Part model, mm, in its own coordinate system. Face numbers are marked on the shaded views. A direction names the side the tool comes from. Round coordinates to 2 decimals unless told otherwise and drop trailing zeros. Write each loop counter-clockwise with the first axis right and the second up, starting at its lowest first coordinate (ties: lowest second). Pieces come first, ordered by that corner, then holes.
1) Saw through at D-D on z = 0. Count the separate pieces of the cut face and the enclosed holes in it, and give its area (3 significant figures).
2) Flat gauge pins, fed straight in: pin 1 (3 mm diameter, centred on x = 20.5, z = -12, fed in from +Y); pin 2 (9.5 mm diameter, centred on x = 39, z = 0, fed in from +Y); pin 3 (8 mm diameter, centred on x = -6.5, z = 16, fed in from +Y); pin 4 (1 mm diameter, centred on y = -10, z = -17.5, fed in from +X). Where does each tip first touch, or does it go through?
3) Saw through at C-C on y = -13.5. Write the cut outline in (x, z).
4) Saw through at A-A on x = 0. Write the cut outline in (y, z) (3 decimals).
5) Which spindle directions (+Z, -Z, +X, -X, +Y, -Y) get a long thin tool onto all of the face, cutting with end or side? Do the marked faces 1, 2, 3 and 4. Say none if no direction does.
6) Pull direction Z, two halves, no side cores. Call the marked faces 5, 6 and 7: +Z half, -Z half, draft (parallel to the pull), parting line (faces both ways), or undercut.
7) Saw through at B-B on y = -5.5. Write the cut outline in (x, z).
8) Drill centre lines: L1, parallel to X at y = -4, z = 0; L2, parallel to Z at x = 0, y = 9; L3, parallel to Z at x = 0, y = -3. Where is each one in solid material? Low to high.
```python
from build123d import *

# Parameters (mm, degrees)
BOSS_EXTRUDE1_DEPTH = 23
CUT_EXTRUDE1_DEPTH  = 46
SKETCH4_R           = 6
CUT_EXTRUDE2_DEPTH  = 46
CUT_EXTRUDE3_DEPTH  = 46
SKETCH6_R           = 4
CUT_EXTRUDE4_DEPTH  = 16
SKETCH7_R           = 3
CUT_EXTRUDE5_DEPTH  = 71.608515808


with BuildPart() as part:
    # Sketch1 → Boss-Extrude1 (new, symmetric)
    with BuildSketch(Plane.XY):
        with BuildLine():
            Line((-54, 3.825), (-30.877783275, 3.825))
            ThreePointArc((-30.877783275, 3.825), (0, 15.075), (30.877783275, 3.825))
            Line((30.877783275, 3.825), (54, 3.825))
            Line((54, 3.825), (54, -8.175))
            Line((54, -8.175), (28, -8.175))
            Line((28, -8.175), (28, -24.175))
            Line((28, -24.175), (22.348098353, -24.175))
            ThreePointArc((22.348098353, -24.175), (0, -8.925), (-22.348098353, -24.175))
            Line((-22.348098353, -24.175), (-28, -24.175))
            Line((-28, -24.175), (-28, -8.175))
            Line((-28, -8.175), (-54, -8.175))
            Line((-54, -8.175), (-54, 3.825))
        make_face()
    extrude(amount=BOSS_EXTRUDE1_DEPTH, both=True)

    # Sketch2 → Cut-Extrude1 (cut)
    with BuildSketch(Plane(origin=(0, 3.825, 0), x_dir=(1, 0, 0), z_dir=(0, 1, 0))):
        with BuildLine():
            ThreePointArc((48.856934001, -23), (54, 0), (48.856934001, 23))
            Line((48.856934001, 23), (54, 23))
            Line((54, 23), (85.001299568, 23))
            Line((85.001299568, 23), (85.001299568, -23))
            Line((85.001299568, -23), (54, -23))
            Line((54, -23), (48.856934001, -23))
        make_face()
        with BuildLine():
            Line((-48.856934001, 23), (-68.265292399, 23))
            Line((-68.265292399, 23), (-68.265292399, -23))
            Line((-68.265292399, -23), (-54, -23))
            Line((-54, -23), (-48.856934001, -23))
            ThreePointArc((-48.856934001, -23), (-54, 0), (-48.856934001, 23))
        make_face()
    extrude(amount=-CUT_EXTRUDE1_DEPTH, mode=Mode.SUBTRACT)

    # Sketch4 → Cut-Extrude2 (cut)
    with BuildSketch(Plane(origin=(0, 3.825, 0), x_dir=(1, 0, 0), z_dir=(0, 1, 0))):
        with Locations(Location((-39, 0, 0), (0, 0, 270))):
            Circle(SKETCH4_R)
        with Locations(Location((39, 0, 0), (0, 0, 270))):
            Circle(SKETCH4_R)
    extrude(amount=-CUT_EXTRUDE2_DEPTH, mode=Mode.SUBTRACT)

    # Sketch5 → Cut-Extrude3 (cut)
    with BuildSketch(Plane(origin=(0, 3.825, 0), x_dir=(1, 0, 0), z_dir=(0, 1, 0))):
        with BuildLine():
            Line((-30.877783275, 13.785122251), (-30.877783275, -13.785122251))
            ThreePointArc((-30.877783275, -13.785122251), (-23, 0), (-30.877783275, 13.785122251))
        make_face()
        with BuildLine():
            Line((30.877783275, 13.785122251), (30.877783275, -13.785122251))
            ThreePointArc((30.877783275, -13.785122251), (23, 0), (30.877783275, 13.785122251))
        make_face()
    extrude(amount=CUT_EXTRUDE3_DEPTH, mode=Mode.SUBTRACT)

    # Sketch6 → Cut-Extrude4 (cut)
    with BuildSketch(Plane(origin=(0, 15.075, 0), x_dir=(1, 0, 0), z_dir=(0, 1, 0))):
        with Locations(Location((0, 0, 0), (0, 0, 270))):
            Circle(SKETCH6_R)
    extrude(amount=-CUT_EXTRUDE4_DEPTH, mode=Mode.SUBTRACT)

    # Sketch7 → Cut-Extrude5 (cut, through all)
    with BuildSketch(Plane(origin=(0, 15.075, 0), x_dir=(1, 0, 0), z_dir=(0, 1, 0))):
        with Locations(Location((0, 0, 0), (0, 0, 270))):
            Circle(SKETCH7_R)
    extrude(amount=-CUT_EXTRUDE5_DEPTH, mode=Mode.SUBTRACT)


solid = part.part
```
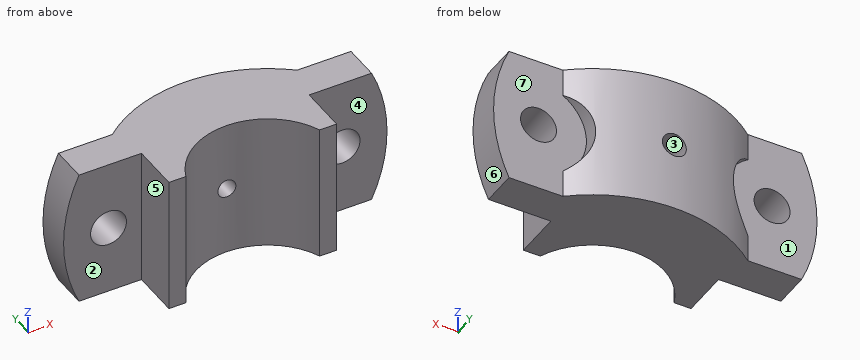
Completed:
1. separate pieces: 4
1. enclosed holes: 0
1. area: 1,660 mm2
2. pin 1: stops at y = 11.15
2. pin 2: passes through
2. pin 3: stops at y = 15.01
2. pin 4: stops at x = 28
3. outline: (-28, -23) - (-14.1, -23) - (-14.1, 23) - (-28, 23) - close; (14.1, -23) - (28, -23) - (28, 23) - (14.1, 23) - close
4. outline: (-8.925, -23) - (15.075, -23) - (15.075, -4) - (-0.925, -4) - (-0.925, -3) - (-8.925, -3) - close; (-8.925, 3) - (-0.925, 3) - (-0.925, 4) - (15.075, 4) - (15.075, 23) - (-8.925, 23) - close
5. face 1: -X, +Y
5. face 2: +Z, -Z, -X, -Y
5. face 3: +Y
5. face 4: +Z, -Z, +X, -Y
6. face 5: draft
6. face 6: parting line
6. face 7: undercut
7. outline: (-48.86, -23) - (48.86, -23) arc R54 ccw to (48.86, 23) - (-48.86, 23) arc R54 ccw to start; hole circle Ø12 at (-39, 0); hole circle Ø6 at (0, 0); hole circle Ø12 at (39, 0)
8. L1: x = -54 to -45, -33 to -3, 3 to 33, 45 to 54
8. L2: z = -23 to -4, 4 to 23
8. L3: z = -23 to -3, 3 to 23
